Could you check a few things on this model? Use its own coordinates, in mm. Face numbers are marked on the shaded views. A direction names the side the tool comes from. Give positions to 0.01 mm unless a question says otherwise; leave off trailing zeros. Order: outer loops, then holes, each group sorted by start corner. A loop starts at its lowest first (then second) coordinate and runs counter-clockwise, first axis right, second up. Notation, with made-up numbers: (67.5, 7) -> (108.5, 7) arc R7 ccw to (108.5, 17) -> close; hole circle Ø8 at (-12, 79). An arc over 180 degrees is marked (long way). Answer as CSV lines item,"result". Start each with the question number.
(1) I want a section at B-B (y = -1.75). Please give me the cut outline in (x, z), plus the area to 3 significant figures.
(2) On a 3-axis mill with a long thin cutter (end or side, diameter ignored), from which of +Z, -Z, +X, -X, +Y, -Y can I reach the whole of each face in a straight line? I mean the marked faces 4 and 5. Say none if no direction works.
(3) I need wall thicknesses on L1, parallel to Z at x = 0, y = -5.5; L2, parallel to Z at x = -2, y = 5.75; L3, parallel to X at y = 2, z = -2.25. Which ranges of each line are inside material? Lowest first, please.
(4) Will these pins go through, and if not, where does the flat tip stop? pin 1 Ø3 at (x, y) = (-1, 6.5) entering from +Z; pin 2 Ø1.5 at (y, z) = (-4, -2) entering from +X; pin 3 Ø0.8 at (y, z) = (9, 2.5) entering from -X.
(5) I want a section at A-A (y = 7.75). Please give me the cut outline in (x, z), plus the area to 3 significant figures.
(6) We'd pull the mould along X, two halves only. Please class the marked faces 1, 2 and 3: released by +X, released by -X, zero draft, split by the parting line, or undercut.
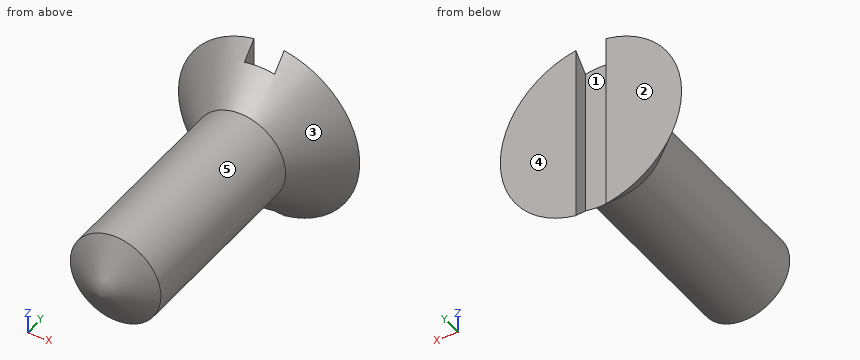
```python
from build123d import *

# Parameters (mm, degrees)
SKETCH2_R           = 3
BOSS_EXTRUDE1_DEPTH = 6.5
SKETCH7_W           = 2
SKETCH7_H           = 1
CUT_EXTRUDE1_DEPTH  = 7


with BuildPart() as part:
    # Sketch2 → Boss-Extrude1 (new body, symmetric)
    with BuildSketch(Plane(origin=(0, 0, 0), x_dir=(1, 0, 0), z_dir=(0, 1, 0))):
        Circle(SKETCH2_R)
    extrude(amount=BOSS_EXTRUDE1_DEPTH, both=True)

    # Sketch5 → Revolve2 (revolve)
    with BuildSketch(Plane.XY):
        Polygon((-3, -6.5), (0, -8.232050808), (0, -6.5), align=None)
    revolve(axis=Axis((0, -6.5, 0), (0, -1, 0)))

    # Sketch6 → Revolve3 (revolve)
    with BuildSketch(Plane.XY):
        Polygon((3, 6.5), (0, 6.5), (0, 9.5), (6, 9.5), align=None)
    revolve(axis=Axis((0, 6.5, 0), (0, 1, 0)))

    # Sketch7 → Cut-Extrude1 (cut, symmetric)
    with BuildSketch(Plane.XY):
        with Locations((0, 9)):
            Rectangle(SKETCH7_W, SKETCH7_H)
    extrude(amount=CUT_EXTRUDE1_DEPTH, both=True, mode=Mode.SUBTRACT)


solid = part.part
```
Final values:
1,outline,"circle Ø6 at (0, 0)"
1,area,"28.3 mm²"
2,face 4,"+Z, -Z, +X, -X, +Y"
2,face 5,"-Y"
3,L1,"-3 to 3"
3,L2,"-2.24 to 2.24"
3,L3,"-1.98 to 1.98"
4,pin 1,"z = 4.42"
4,pin 2,"x = 2.73"
4,pin 3,"x = -5.38"
5,outline,"circle Ø8.5 at (0, 0)"
5,area,"56.7 mm²"
6,face 1,"undercut"
6,face 2,"zero draft"
6,face 3,"split by the parting line"
